Input: dimensioned drawing with shaded views. Units: mm. Origin: part minimum x, y, z. A direction names the side the tool comes from. Coordinates: 2 decimals unless noted, no trailing zeros. Loops run counter-clockwise (first coordinate to the right, second up) from the corner with the lowest first, then second, coordinate; pieces in that order, holes last.
Item 1: Section query B-B, the plane x = 31. Return the cut outline in (y, z), then the cut area to 3 significant figures.
Item 2: Section query D-D, the plane y = 23. State how many separate pieces and enclosed holes the cut face has.
Item 3: Pull-direction query (X, two-part tool) for the marked faces 3, 4 and 5; classes: +X half, -X half, draft (parallel to the pull), parting line (faces both ways), or undercut.
Item 4: Reachability of the marked faces 1 and 2 from +Z, -Z, +X, -X, +Y, -Y: full face, straight path, thin tool, end or side. Return the list, or none.
Item 5: Pin query (flat end, axial travel): pin 1 Ø10.5 at (x, z) = (15, 16.5) entering from +Y; pin 2 Ø1.6 at (x, z) = (4.29, 30.76) entering from +Y. Return the tip coordinate at first contact, or that it passes through.
Item 6: Section query C-C, the plane z = 11. Return the cut outline in (x, y), then the cut area to 3 significant figures.
Item 7: Line query: probe 1 along X at (y, z) = (9.5, 19); probe 2 along Z at (x, y) = (24.5, 19.75); probe 3 along Y at (x, z) = (22.5, 16). Output: solid intervals per line, ascending.
Item 8: Section query A-A, the plane y = 10.75. Return the cut outline in (x, z).
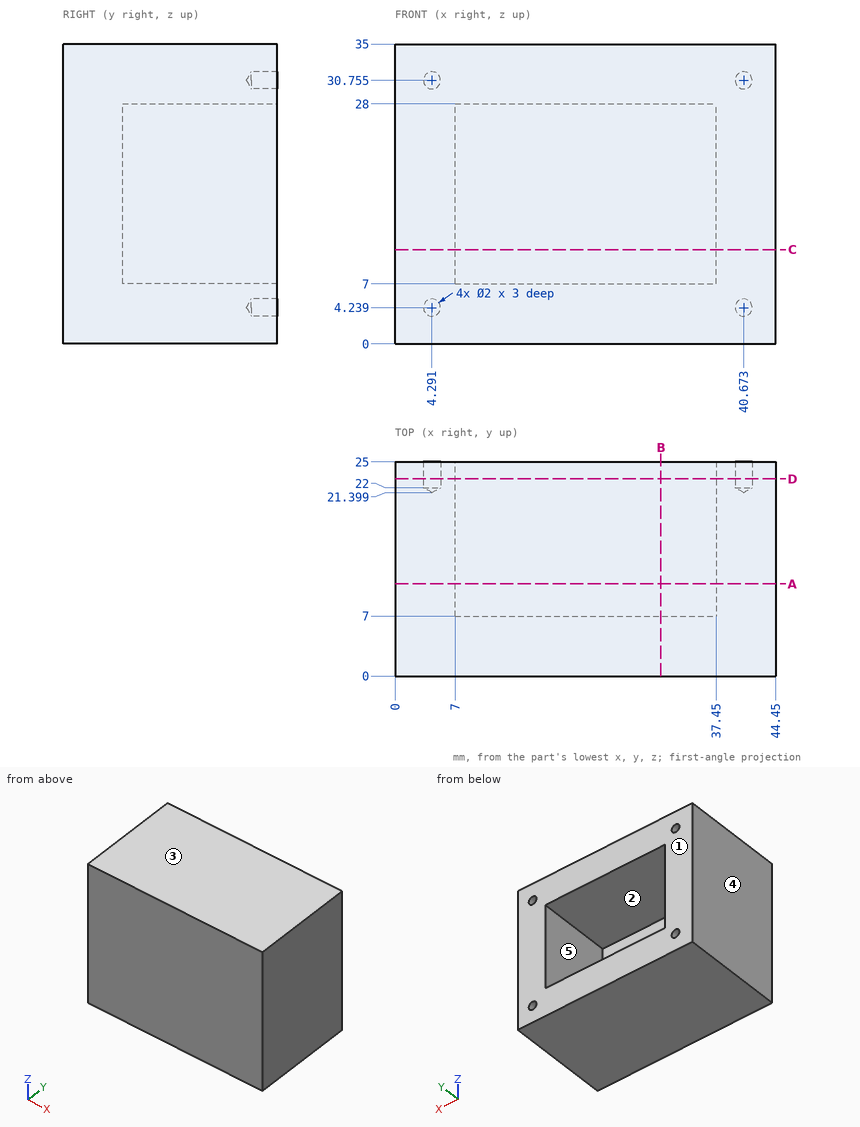
Verdict:
1. outline: (0, 0) - (25, 0) - (25, 7) - (7, 7) - (7, 28) - (25, 28) - (25, 35) - (0, 35) - close
1. area: 497 mm2
2. separate pieces: 1
2. enclosed holes: 5
3. face 3: draft
3. face 4: -X half
3. face 5: undercut
4. face 1: +Z, -Z, +X, -X, +Y
4. face 2: +Y
5. pin 1: stops at y = 7
5. pin 2: stops at y = 21.88
6. outline: (0, 0) - (44.45, 0) - (44.45, 25) - (37.45, 25) - (37.45, 7) - (7, 7) - (7, 25) - (0, 25) - close
6. area: 563 mm2
7. probe 1: x = 0 to 7, 37.45 to 44.45
7. probe 2: z = 0 to 7, 28 to 35
7. probe 3: y = 0 to 7
8. outline: (0, 0) - (44.45, 0) - (44.45, 35) - (0, 35) - close; hole (7, 7) - (37.45, 7) - (37.45, 28) - (7, 28) - close
